from build123d import *

# Parameters (mm, degrees)
F1_START       = 19.05
F1_DEPTH       = 31.75
F3_DEPTH       = 12.7
F5_DEPTH       = 25.4
F7_DEPTH       = 50.8
F10_T4_DEPTH   = 118.8107467306
F10_T9_DEPTH   = 118.8107467306
F11_W          = 5.588
F11_H          = 36.83
F11_H_2        = 36.322
F12_DEPTH      = 25.4
F12_DEPTH_BACK = 19.05
F13_W          = 26.0096
F13_H          = 3.048
F14_DEPTH      = 19.05
F15_W          = 26.0096
F15_H          = 3.048
F15_W_2        = 25.684906454
F16_DEPTH      = 25.4
F17_R          = 34.3708732133
F18_DEPTH      = 63.5
F19_W          = 101.6
F19_H          = 32.0445634425
F19_W_2        = 28.5529913381
F19_H_2        = 6.6054575145
F19_H_3        = 10.527446866
F19_W_3        = 20.7230086619
F19_H_4        = 8.6696632206
F19_H_5        = 7.8439861536
F20_DEPTH      = 38.1
F21_SIZE       = 5.08


# Not quite as in the source:
# - a fillet or chamfer that OpenCascade refuses, or shapes differently, is made with other operations: its cross-section is extruded or revolved along the edge and cut away or added
# - a feature of the source that left no trace in its solid (it failed there, or was rolled back) is left out


with BuildPart() as f1:
    # F0 (on Top) → F1 (new body)
    with BuildSketch(Plane.XY.offset(F1_START)):
        Polygon((-27.681270317, -38.1), (-23.1827056925, -38.1), (-29.0714032363, -33.8216107999), align=None)
        Polygon((-29.0714032363, -33.8216107999), (-23.1827056925, -38.1), (23.1827056925, -38.1), (29.0714032363, -33.8216107999), (43.3991033054, 10.2745158286), (41.1498209932, 17.1970949714), (3.6394152315, 44.45), (-3.6394152315, 44.45), (-41.1498209932, 17.1970949714), (-43.3991033054, 10.2745158286), align=None)
        with BuildLine():
            Line((23.1827056925, -38.1), (-23.1827056925, -38.1))
            Line((-23.1827056925, -38.1), (-27.681270317, -38.1))
            ThreePointArc((-27.681270317, -38.1), (0, -47.0941899427), (27.681270317, -38.1))
            Line((27.681270317, -38.1), (23.1827056925, -38.1))
        make_face()
        Polygon((-37.8114284312, -27.4716107999), (-29.0714032363, -33.8216107999), (-43.3991033054, 10.2745158286), (-46.7374958674, 0), align=None)
        Polygon((29.0714032363, -33.8216107999), (23.1827056925, -38.1), (27.681270317, -38.1), align=None)
        Polygon((-44.7892362247, 14.5529050286), (-43.3991033054, 10.2745158286), (-41.1498209932, 17.1970949714), align=None)
        Polygon((43.3991033054, 10.2745158286), (29.0714032363, -33.8216107999), (37.8114284312, -27.4716107999), (46.7374958674, 0), align=None)
        with BuildLine():
            Line((-44.7892362247, 14.5529050286), (-41.1498209932, 17.1970949714))
            Line((-41.1498209932, 17.1970949714), (-3.6394152315, 44.45))
            Line((-3.6394152315, 44.45), (0, 47.0941899427))
            ThreePointArc((0, 47.0941899427), (-27.681270317, 38.1), (-44.7892362247, 14.5529050286))
        make_face()
        Polygon((41.1498209932, 17.1970949714), (43.3991033054, 10.2745158286), (44.7892362247, 14.5529050286), align=None)
        Polygon((0, 47.0941899427), (-3.6394152315, 44.45), (3.6394152315, 44.45), align=None)
        with BuildLine():
            ThreePointArc((44.7892362247, 14.5529050286), (27.681270317, 38.1), (0, 47.0941899427))
            Line((0, 47.0941899427), (3.6394152315, 44.45))
            Line((3.6394152315, 44.45), (41.1498209932, 17.1970949714))
            Line((41.1498209932, 17.1970949714), (44.7892362247, 14.5529050286))
        make_face()
    extrude(amount=F1_DEPTH)

    # F2 (on Right) → F3 (cut, symmetric)
    with BuildSketch(Plane.YZ):
        Polygon((-44.8449260175, 25.4), (69.4550739825, 57.15), (-44.8449260175, 57.15), align=None)
    extrude(amount=F3_DEPTH, both=True, mode=Mode.SUBTRACT)

    # F4 (on Right) → F5 (cut, symmetric)
    with BuildSketch(Plane.YZ):
        Polygon((-44.8449260175, 31.75), (70.0721293688, 57.15), (-44.8449260175, 57.15), align=None)
    extrude(amount=F5_DEPTH, both=True, mode=Mode.SUBTRACT)

    # F6 (on Right) → F7 (cut, symmetric)
    with BuildSketch(Plane.YZ):
        Polygon((69.4550739825, 57.15), (-44.8449260175, 57.15), (-44.8449260175, 38.1), (5.1235620631, 46.4280813468), (48.464309937, 53.6515393258), align=None)
        Polygon((48.464309937, 46.4280813468), (48.464309937, 53.6515393258), (5.1235620631, 46.4280813468), align=None)
    extrude(amount=F7_DEPTH, both=True, mode=Mode.SUBTRACT)

    # F10: fillet of radius 5.08 on 2 edges, made by hand


with BuildPart() as f10_tool2:
    # F10_s3 → F10_t4 (new body)
    with BuildSketch(Plane(origin=(0, -48.4660281995, -10.712396973), x_dir=(1, 0, 0), z_dir=(0, 0.9764331595, 0.2158200292))):
        with BuildLine():
            ThreePointArc((-12.7, -35.6001860579), (-14.1878975516, -39.1922885063), (-17.78, -40.6801860579))
            Line((-17.78, -40.6801860579), (-12.7, -40.6801860579))
            Line((-12.7, -40.6801860579), (-12.7, -35.6001860579))
        make_face()
    extrude(amount=F10_T4_DEPTH)

    split(bisect_by=Plane(origin=(0, -9.762530517, 35.1451098613), x_dir=(1, 0, 0), z_dir=(0, -0.2676438638, 0.9635179096)), keep=Keep.TOP)


with BuildPart() as f1_1:
    add(f1.part)

    # F10_t1: cut F10_tool2
    add(f10_tool2.part, mode=Mode.SUBTRACT)


with BuildPart() as f10_tool7:
    # F10_s8 → F10_t9 (new body)
    with BuildSketch(Plane(origin=(0, -48.4660281995, -10.712396973), x_dir=(1, 0, 0), z_dir=(0, 0.9764331595, 0.2158200292))):
        with BuildLine():
            ThreePointArc((17.78, -40.6801860579), (14.1878975516, -39.1922885063), (12.7, -35.6001860579))
            Line((12.7, -35.6001860579), (12.7, -40.6801860579))
            Line((12.7, -40.6801860579), (17.78, -40.6801860579))
        make_face()
    extrude(amount=F10_T9_DEPTH)

    split(bisect_by=Plane(origin=(0, -9.762530517, 35.1451098613), x_dir=(1, 0, 0), z_dir=(0, -0.2676438638, 0.9635179096)), keep=Keep.TOP)


with BuildPart() as f1_2:
    add(f1_1.part)

    # F10_t6: cut F10_tool7
    add(f10_tool7.part, mode=Mode.SUBTRACT)

    # F11 (on offset) → F12 (cut, two sides)
    with BuildSketch(Plane.XY.offset(50.8)) as f12_sk:
        with Locations((-33.274, -0.7722239547)):
            Rectangle(F11_W, F11_H)
        with Locations((-22.606, 3.0599313468)):
            Rectangle(F11_W, F11_H_2)
        with Locations((33.274, 0.82358277)):
            Rectangle(F11_W, F11_H_2)
        with Locations((22.606, 3.0599313468)):
            Rectangle(F11_W, F11_H_2)
    extrude(amount=F12_DEPTH, mode=Mode.SUBTRACT)
    extrude(f12_sk.sketch, amount=-F12_DEPTH_BACK, mode=Mode.SUBTRACT)

    # F13 (on offset) → F14 (cut)
    with BuildSketch(Plane.XY.offset(50.8)):
        with Locations((0, 12.1964783492)):
            Rectangle(F13_W, F13_H)
        with Locations((0, 28.4524783492)):
            Rectangle(F13_W, F13_H)
        with Locations((0, 20.3244783492)):
            Rectangle(F13_W, F13_H)
    extrude(amount=-F14_DEPTH, mode=Mode.SUBTRACT)

    # F15 (on offset) → F16 (cut)
    with BuildSketch(Plane.XY.offset(50.8)):
        with Locations((0, -4.0595216508)):
            Rectangle(F15_W, F15_H)
        with Locations((0.0519962238, -12.1875216508)):
            Rectangle(F15_W_2, F15_H)
        with Locations((0, 4.0684783492)):
            Rectangle(F15_W, F15_H)
    extrude(amount=-F16_DEPTH, mode=Mode.SUBTRACT)

    # F17 (on Right) → F18 (cut, symmetric)
    with BuildSketch(Plane.YZ):
        with Locations((0, 75.4981189966)):
            Circle(F17_R)
    extrude(amount=F18_DEPTH, both=True, mode=Mode.SUBTRACT)

    # F19 (on offset) → F20 (cut, symmetric)
    with BuildSketch(Plane.XY.offset(50.8)):
        with Locations((-3.9149913381, -37.4202784151)):
            Rectangle(F19_W, F19_H)
        Polygon((46.8850086619, 51.8795326352), (-54.7149913381, 51.8795326352), (-54.7149913381, 33.7145216763), (-48.3649913381, 33.7145216763), (-48.3649913381, 40.3199791908), (-19.812, 40.3199791908), (-19.812, 33.7145216763), (19.812, 33.7145216763), (19.812, 41.5585078299), (40.5350086619, 41.5585078299), (40.5350086619, 33.7145216763), (46.8850086619, 33.7145216763), align=None)
        with Locations((-34.088495669, 37.0172504336)):
            Rectangle(F19_W_2, F19_H_2)
        with Locations((-34.088495669, 28.4507982433)):
            Rectangle(F19_W_2, F19_H_3)
        with Locations((30.173504331, 29.379690066)):
            Rectangle(F19_W_3, F19_H_4)
        with Locations((30.173504331, 37.6365147531)):
            Rectangle(F19_W_3, F19_H_5)
    extrude(amount=F20_DEPTH, both=True, mode=Mode.SUBTRACT)

    # F21
    f21_edges = [f1_2.edges().sort_by_distance(p)[0] for p in [
        (-19.812, 33.714522, 32.739041),
        (19.812, 33.714522, 32.739041),
    ]]
    chamfer(f21_edges, length=F21_SIZE)


solid = f1_2.part
Input: part model. Units: mm. Frame: model coordinates. A direction names the side the tool comes from. Give positions to 0.01 mm unless a question says otherwise; leave off trailing zeros. Order: outer loops, then holes, each group sorted by start corner. A loop starts at its lowest first (then second) coordinate and runs counter-clockwise, first axis right, second up. Notation, with made-up numbers: (4, -25.75) -> (49, -25.75) arc R19 ccw to (49, 4.25) -> close; hole circle Ø9 at (36, 20.25). An arc over 180 degrees is marked (long way). Use one line per item in the form item = value.
1) First-contact query: pin 1 Ø1.7 at (x, z) = (-23.5, 36) entering from +Y; pin 2 Ø4 at (x, y) = (-21.5, -12.5) entering from +Z; pin 3 Ø3.5 at (y, z) = (20.5, 40.5) entering from -X. Flat tips, straight axial feed; report the tip coordinate or a pass-through.
Response values:
pin_1 = 23.19
pin_2 = 39.14
pin_3 = -43.2
2) Mould query, pull axis Y, two halves, no side actions, for faces 1 (the flat face through (13.005, 28, 39)), 2 (the flat face through (0.2, 31.1, 46.428)), 3 (the flat face through (20.797, -16.179, 38.086)). Classes: pulls with the +Y half, pulls with the -Y half, needs draft (parallel to the pull), parting line crosses it, or undercut.
Response values:
face_1 = undercut
face_2 = needs draft
face_3 = pulls with the -Y half
3) Reachability of faces 4 (the flat face through (-17.236, 31.21, 32.547)), 5 (the flat face through (19.35, 19.345, 45.938)), 6 (the flat face through (-45.045, 5.209, 30.709)), 7 (the flat face through (23, 3, 31.75)) from +Z, -Z, +X, -X, +Y, -Y: full face, straight path, thin tool, end or side. Return the list, or none.
Response values:
face_4 = +Z, -Z, -X, +Y
face_5 = +Z, -Y
face_6 = +Z, -Z, -X
face_7 = +Z
4) Section D-D, the plane x = 23. Return loops of the section in (y, z).
Response values:
outline = (-21.4, 19.05) -> (25.04, 19.05) -> (25.04, 46.43) -> (21.56, 46.43) -> (21.22, 46.35) -> (21.22, 31.75) -> (-15.1, 31.75) -> (-15.1, 38.32) -> (-21.4, 36.93) -> close
5) Line query: probe 1 along Y at (x, z) = (10, 30.5); probe 2 along Y at (x, z) = (-5, 36.5); probe 3 along X at (y, z) = (14.5, 37). Output: solid intervals per line, ascending.
Response values:
probe_1 = -21.4 to -13.71, -10.66 to -5.58, -2.54 to 2.54, 5.59 to 33.71
probe_2 = -2.54 to 2.54, 5.59 to 10.67, 13.72 to 18.8, 21.85 to 26.93, 29.98 to 33.71
probe_3 = -44.77 to -36.07, -30.48 to -25.4, -19.81 to 19.81, 25.4 to 30.48, 36.07 to 44.77
6) Section B-B, the plane x = 33. Return loops of the section in (y, z), and give its area (3 significant figures).
Response values:
outline = (-21.4, 19.05) -> (25.04, 19.05) -> (25.04, 46.43) -> (18.98, 46.43) -> (18.98, 31.75) -> (-17.34, 31.75) -> (-17.34, 42.68) -> (-21.4, 42.01) -> close
area = 722 mm^2
7) Section C-C, the plane z = 21.25. Return loops of the section in (x, y), and give its area (3 significant figures).
Response values:
outline = (-46.74, 0) -> (-39.78, -21.4) -> (39.78, -21.4) -> (46.74, 0) -> (43.4, 10.27) -> (44.79, 14.55) arc R47.09 ccw to (39.88, 25.04) -> (19.81, 25.04) -> (19.81, 28.63) -> (14.73, 33.71) -> (-14.73, 33.71) -> (-19.81, 28.63) -> (-19.81, 23.19) -> (-40.99, 23.19) arc R47.09 ccw to (-44.79, 14.55) -> (-43.4, 10.27) -> close
area = 4,330 mm^2
8) Section A-A, the plane z = 29.25. Return loops of the section in (x, y), and give its area (3 significant figures).
Response values:
outline = (-46.74, 0) -> (-39.78, -21.4) -> (39.78, -21.4) -> (46.74, 0) -> (43.4, 10.27) -> (44.79, 14.55) arc R47.09 ccw to (39.88, 25.04) -> (19.81, 25.04) -> (19.81, 28.63) -> (14.73, 33.71) -> (-14.73, 33.71) -> (-19.81, 28.63) -> (-19.81, 23.19) -> (-40.99, 23.19) arc R47.09 ccw to (-44.79, 14.55) -> (-43.4, 10.27) -> close; hole (-13, -5.58) -> (13, -5.58) -> (13, -2.54) -> (-13, -2.54) -> close; hole (-13, 2.54) -> (13, 2.54) -> (13, 5.59) -> (-13, 5.59) -> close; hole (-12.79, -13.71) -> (12.89, -13.71) -> (12.89, -10.66) -> (-12.79, -10.66) -> close
area = 4,090 mm^2
